Could you check a few things on this model? Use its own coordinates, in mm. A direction names the side the tool comes from. Give positions to 0.01 mm unless a question says otherwise; leave off trailing zeros. Order: outer loops, then holes, each group sorted by start corner. A loop starts at its lowest first (then second) coordinate and runs counter-clockwise, first axis right, second up. Notation, with made-up numbers: (-31, -13.75) - (-15, -13.75) arc R23 cw to (-15, 15.25) - close; hole circle Ø1 at (49, 3.5). An arc over 180 degrees is marked (long way). Put each result on its own line as item: value.
from build123d import *

# Parameters (mm, degrees)
SKETCH1_W           = 304.8
SKETCH1_H           = 152.4
BOSS_EXTRUDE1_DEPTH = 304.8
SHELL1_T            = -9.525
BOSS_EXTRUDE2_DEPTH = 2.54
SKETCH4_R           = 47.625
CUT_EXTRUDE1_DEPTH  = 7.62


with BuildPart() as part:
    # Sketch1 → Boss-Extrude1 (new body)
    with BuildSketch(Plane.XY):
        Rectangle(SKETCH1_W, SKETCH1_H)
    extrude(amount=BOSS_EXTRUDE1_DEPTH)

    # Shell1
    shell1_openings = [part.faces().sort_by_distance(p)[0] for p in [
        (0, 0, 304.8),
        (0, 76.2, 152.4),
    ]]
    offset(amount=SHELL1_T, openings=shell1_openings, kind=Kind.INTERSECTION)

    # Sketch2 → Boss-Extrude2 (add)
    with BuildSketch(Plane(origin=(0, 76.2, 0), x_dir=(1, 0, 0), z_dir=(0, 1, 0))):
        Polygon((-142.875, -304.8), (142.875, -304.8), (152.4, -304.8), (152.4, 0), (-152.4, 0), (-152.4, -304.8), align=None)
    extrude(amount=BOSS_EXTRUDE2_DEPTH)

    # Sketch4 → Cut-Extrude1 (cut)
    with BuildSketch(Plane(origin=(0, 78.74, 0), x_dir=(1, 0, 0), z_dir=(0, 1, 0))):
        with Locations((15.875, -155.428881859)):
            Circle(SKETCH4_R)
    extrude(amount=-CUT_EXTRUDE1_DEPTH, mode=Mode.SUBTRACT)


solid = part.part
1) Suppose I cut it at B-B, the plane z = 22. List the corners of the cut face in (x, y) for me (3 decimals).
Filled in:
outline: (-152.4, -76.2) - (152.4, -76.2) - (152.4, 78.74) - (-152.4, 78.74) - close; hole (-142.875, -66.675) - (142.875, -66.675) - (142.875, 76.2) - (-142.875, 76.2) - close
2) We'd pull the mould along X, two halves only. Please class faces 1 (the flat face through (-34, 76.2, 155)), 2 (the flat face through (-12, -68, 304.8)), 3 (the flat face through (-152.4, 0, 150)): pulls with the +X half, pulls with the -X half, needs draft (parallel to the pull), parting line crosses it, or undercut.
Filled in:
face 1: undercut
face 2: needs draft
face 3: pulls with the -X half
3) If I drill on line 1 (X direction, y = 23.5, z = 271.5) (3 decimals); line 2 (Y direction, x = -71.5, z = 25.5) (3 decimals); line 3 (Z direction, x = 110, y = -7) (3 decimals), over which ranges is the centre line in solid material (lowest first)? Write a range as [from, to].
Filled in:
line 1: x = [-152.4, -142.875], [142.875, 152.4]
line 2: y = [-76.2, -66.675], [76.2, 78.74]
line 3: z = [0, 9.525]
4) I'm going to push a flat-ended pin straight in: pin 1 (1.5 mm diameter, centred on x = 76.5, y = -49.5, fed in from +Z) (3 decimals). Where does the tip first touch, or does it pass through?
Filled in:
pin 1: stops at z = 9.525
5) Suppose I cut it at D-D, the plane y = 26. List the corners of the cut face in (x, z) for me (3 decimals), and give its area (3 significant figures).
Filled in:
outline: (-152.4, 0) - (152.4, 0) - (152.4, 304.8) - (142.875, 304.8) - (142.875, 9.525) - (-142.875, 9.525) - (-142.875, 304.8) - (-152.4, 304.8) - close
area: 8,530 mm^2
6) Suppose I cut it at A-A, the plane x = -66. List the corners of the cut face in (y, z) for me (3 decimals), and give its area (3 significant figures).
Filled in:
outline: (-76.2, 0) - (78.74, 0) - (78.74, 304.8) - (76.2, 304.8) - (76.2, 9.525) - (-66.675, 9.525) - (-66.675, 304.8) - (-76.2, 304.8) - close
area: 5,040 mm^2
7) Suppose I cut it at C-C, the plane x = 51. List the corners of the cut face in (y, z) for me (3 decimals), and give its area (3 significant figures).
Filled in:
outline: (-76.2, 0) - (78.74, 0) - (78.74, 123.267) - (76.2, 123.267) - (76.2, 9.525) - (-66.675, 9.525) - (-66.675, 304.8) - (-76.2, 304.8) - close; (76.2, 187.591) - (78.74, 187.591) - (78.74, 304.8) - (76.2, 304.8) - close
area: 4,870 mm^2
8) Which directions (+Z, -Z, +X, -X, +Y, -Y) give clear straight access to the entire face, cutting with the end or side of a thin tool? Please do faces 4 (the flat face through (-142.875, 4, 155)), 5 (the cylindrical face through (37.85, 77.49, 197.68)), 6 (the flat face through (2, 0, 0)).
Filled in:
face 4: +Z
face 5: +Y
face 6: -Z, +X, -X, +Y, -Y
